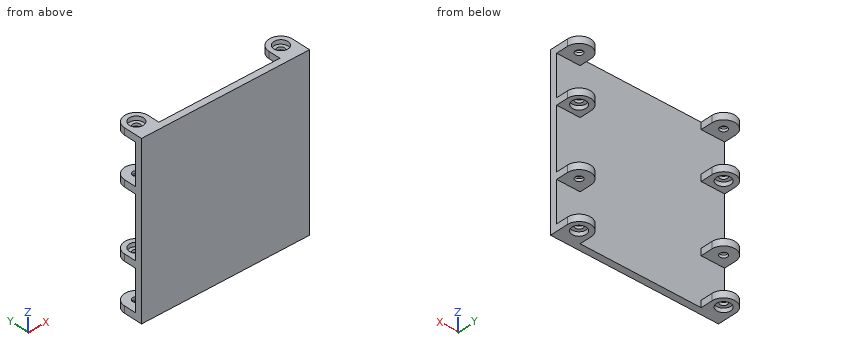
Autodesk Inventor part; units mm, degrees
ref_plane "Work Plane1" through (0, 0, 90) normal (0, 0, 1) x (1, 0, 0)
ref_plane "Work Plane2" through (0, 0, -90) normal (0, 0, 1) x (1, 0, 0)
ref_plane "YZ Plane" through (0, 0, 0) normal (1, 0, 0) x (0, 1, 0)
sketch "Sketch1" plane through (0, 0, 0) normal (0, 0, 1) x (1, 0, 0)
  line L0 (-250, -10) -> (250, -10)
  line L1 (250, -10) -> (250, 10)
  line L2 (250, 10) -> (-250, 10)
  line L3 (-250, 10) -> (-250, -10)
  line L4 (-250, -10) -> (250, 10) construction
  line L5 (250, -10) -> (-250, 10) construction
  point P0 (0, 0)
  dimension "d0" = 500
  dimension "d1" = 20
extrude "Extrusion1" add sketch "Sketch1" along normal mid plane 500
sketch "Sketch2" plane through (0, 0, 250) normal (0, 0, 1) x (1, 0, 0)
  arc A0 (-180, 45) -> (-250, 45) centre (-215, 45) ccw
  line L0 (250, 10) -> (-250, 10) construction
  circle A1 centre (-215, 45) radius 11
  line L1 (-250, 45) -> (-250, 0)
  line L2 (-180, 45) -> (-180, 0)
  line L3 (-180, 0) -> (-250, 0)
  point P0 (0, 0)
  dimension "d4" = 70
  dimension "d5" = 215
  dimension "d6" = 45
  dimension "d7" = 22
  dimension "d9" = 10
extrude "Extrusion2" add sketch "Sketch2" against normal blind 20
ref_plane "Work Plane1" through (0, 0, 90) normal (0, 0, 1) x (1, 0, 0)
sketch "Sketch3" plane through (0, 0, 90) normal (0, 0, 1) x (1, 0, 0)
  arc A0 (-180, 45) -> (-250, 45) centre (-215, 45) ccw construction
  circle A1 centre (-215, 45) radius 11 construction
  line L0 (-180, 45) -> (-180, 10) construction
  line L1 (-250, 45) -> (-250, -10) construction
  circle A2 centre (-215, 45) radius 11
  arc A3 (-180, 45) -> (-250, 45) centre (-215, 45) ccw
  line L2 (-250, 45) -> (-250, 0)
  line L3 (-180, 45) -> (-180, 0)
  line L4 (-180, 0) -> (-250, 0)
  point P0 (0, 0)
extrude "Extrusion3" add sketch "Sketch3" along normal blind 20
sketch "Sketch4" plane through (0, 0, 250) normal (0, 0, 1) x (1, 0, 0)
  circle A0 centre (-215, 45) radius 11 construction
  circle A1 centre (-215, 45) radius 21
  point P0 (0, 0)
  dimension "d15" = 42
extrude "Extrusion4" cut sketch "Sketch4" against normal blind 12
sketch "Sketch5" plane through (0, 0, 90) normal (0, 0, -1) x (-1, 0, 0)
  circle A0 centre (215, 45) radius 11 construction
  circle A1 centre (215, 45) radius 21
  point P0 (0, 0)
  dimension "d18" = 42
extrude "Extrusion5" cut sketch "Sketch5" against normal blind 12
sketch "Sketch6" plane through (0, 0, 250) normal (0, 0, 1) x (1, 0, 0)
  arc A0 (250, 45) -> (180, 45) centre (215, 45) ccw
  circle A1 centre (215, 45) radius 11
  line L0 (180, 45) -> (180, 0)
  line L1 (180, 0) -> (250, 0)
  line L2 (250, 0) -> (250, 45)
  point P0 (0, 0)
  dimension "d21" = 70
  dimension "d22" = 215
  dimension "d23" = 45
  dimension "d24" = 22
  dimension "d25" = 0
extrude "Extrusion6" add sketch "Sketch6" against normal blind 20
sketch "Sketch7" plane through (0, 0, 90) normal (0, 0, 1) x (1, 0, 0)
  arc A0 (250, 45) -> (180, 45) centre (215, 45) ccw construction
  circle A1 centre (215, 45) radius 11 construction
  arc A2 (250, 45) -> (180, 45) centre (215, 45) ccw
  circle A3 centre (215, 45) radius 11
  circle A4 centre (215, 45) radius 11
  line L0 (250, 45) -> (250, 10)
  line L1 (250, 45) -> (250, 0)
  line L2 (250, 0) -> (250, 0)
  arc A5 (250, 45) -> (180, 45) centre (215, 45) ccw
  line L3 (250, 0) -> (250, 45)
  line L4 (180, 45) -> (180, 0)
  line L5 (180, 0) -> (250, 0)
  point P0 (0, 0)
  dimension "d28" = 22
  dimension "d29" = 45
extrude "Extrusion7" add sketch "Sketch7" along normal blind 20
sketch "Sketch8" plane through (0, 0, 250) normal (0, 0, 1) x (1, 0, 0)
  circle A0 centre (215, 45) radius 11 construction
  circle A1 centre (215, 45) radius 21
  point P0 (0, 0)
  dimension "d32" = 42
extrude "Extrusion8" cut sketch "Sketch8" against normal blind 12
sketch "Sketch9" plane through (0, 0, 90) normal (0, 0, -1) x (-1, 0, 0)
  circle A0 centre (-215, 45) radius 11 construction
  circle A1 centre (-215, 45) radius 21
  point P0 (0, 0)
  dimension "d35" = 42
extrude "Extrusion9" cut sketch "Sketch9" against normal blind 12
sketch "Sketch10" plane through (0, 0, -250) normal (0, 0, -1) x (-1, 0, 0)
  arc A0 (-180, 45) -> (-250, 45) centre (-215, 45) ccw construction
  line L0 (-180, 45) -> (-180, 10) construction
  line L1 (-250, 10) -> (-250, 45) construction
  line L2 (250, 10) -> (-250, 10) construction
  circle A1 centre (-215, 45) radius 11 construction
  arc A2 (-180, 45) -> (-250, 45) centre (-215, 45) ccw
  arc A3 (-180, 45) -> (-250, 45) centre (-215, 45) ccw
  circle A4 centre (-215, 45) radius 11
  line L3 (-250, 45) -> (-250, 10)
  line L4 (-250, -10) -> (-250, 45) construction
  line L5 (-180, 10) -> (-180, 45)
  line L6 (-250, 10) -> (-180, 10)
  point P0 (0, 0)
  dimension "d38" = 22
extrude "Extrusion10" add sketch "Sketch10" against normal blind 20
sketch "Sketch11" plane through (0, 0, -250) normal (0, 0, -1) x (-1, 0, 0)
  arc A0 (250, 45) -> (180, 45) centre (215, 45) ccw construction
  circle A1 centre (215, 45) radius 11 construction
  arc A2 (250, 45) -> (180, 45) centre (215, 45) ccw
  arc A3 (250, 45) -> (180, 45) centre (215, 45) ccw
  circle A4 centre (215, 45) radius 11
  line L0 (180, 45) -> (180, 10)
  line L1 (180, 10) -> (250, 10)
  line L2 (180, 45) -> (180, 10)
  line L3 (180, 10) -> (250, 10)
  line L4 (250, 10) -> (250, 45)
  point P0 (0, 0)
  dimension "d41" = 22
extrude "Extrusion11" add sketch "Sketch11" against normal blind 20
ref_plane "Work Plane2" through (0, 0, -90) normal (0, 0, 1) x (1, 0, 0)
sketch "Sketch12" plane through (0, 0, -90) normal (0, 0, 1) x (1, 0, 0)
  arc A0 (250, 45) -> (180, 45) centre (215, 45) ccw construction
  circle A1 centre (215, 45) radius 11 construction
  arc A2 (250, 45) -> (180, 45) centre (215, 45) ccw
  arc A3 (250, 45) -> (180, 45) centre (215, 45) ccw
  circle A4 centre (215, 45) radius 11
  line L0 (250, 10) -> (180, 10)
  line L1 (250, 45) -> (250, 10)
  line L2 (250, 10) -> (180, 10)
  line L3 (180, 10) -> (180, 45)
  point P0 (0, 0)
extrude "Extrusion12" add sketch "Sketch12" against normal blind 20
sketch "Sketch13" plane through (0, 0, -250) normal (0, 0, -1) x (-1, 0, 0)
  circle A0 centre (-215, 45) radius 11 construction
  circle A1 centre (-215, 45) radius 21
  point P0 (0, 0)
  dimension "d47" = 42
extrude "Extrusion13" cut sketch "Sketch13" against normal blind 12
sketch "Sketch14" plane through (0, 0, -90) normal (0, 0, 1) x (1, 0, 0)
  circle A0 centre (215, 45) radius 11 construction
  circle A1 centre (215, 45) radius 21
  point P0 (0, 0)
  dimension "d50" = 42
extrude "Extrusion14" cut sketch "Sketch14" against normal blind 12
sketch "Sketch15" plane through (0, 0, -90) normal (0, 0, 1) x (1, 0, 0)
  arc A0 (-180, 45) -> (-250, 45) centre (-215, 45) ccw
  arc A1 (-180, 45) -> (-250, 45) centre (-215, 45) ccw
  arc A2 (-180, 45) -> (-250, 45) centre (-215, 45) ccw construction
  circle A3 centre (-215, 45) radius 11 construction
  circle A4 centre (-215, 45) radius 11
  line L0 (-180, 45) -> (-180, 10)
  line L1 (-180, 45) -> (-180, 10)
  line L2 (-250, 10) -> (-180, 10)
  line L3 (-180, 10) -> (-250, 10)
  line L4 (-250, 10) -> (-250, 45)
  point P0 (0, 0)
  dimension "d53" = 22
extrude "Extrusion15" add sketch "Sketch15" against normal blind 20
sketch "Sketch16" plane through (0, 0, -250) normal (0, 0, -1) x (-1, 0, 0)
  circle A0 centre (215, 45) radius 11 construction
  circle A1 centre (215, 45) radius 21
  point P0 (0, 0)
  dimension "d56" = 42
extrude "Extrusion16" cut sketch "Sketch16" against normal blind 12
sketch "Sketch17" plane through (0, 0, -90) normal (0, 0, 1) x (1, 0, 0)
  circle A0 centre (-215, 45) radius 11 construction
  circle A1 centre (-215, 45) radius 21
  point P0 (0, 0)
  dimension "d59" = 42
extrude "Extrusion17" cut sketch "Sketch17" against normal blind 12
properties part number "MecanumPlate_FEA" material "Aluminum 6061"
Geometry: final body of the model. Coordinates: model frame, mm. Coordinates: 2 decimals unless noted, no trailing zeros. Order: outer loops, then holes, each group sorted by start corner. A loop starts at its lowest first (then second) coordinate and runs counter-clockwise, first axis right, second up. Notation, with made-up numbers: (15, 35) -> (60, 35) arc R24 cw to (60, 45) -> close; hole circle Ø3 at (-37.75, 40). An arc over 180 degrees is marked (long way). Write each question's results on one line, items separated by ' | '. Start each with the question number.
1) Material intervals for line 1 along Z through (x, y) = (196, 19); line 2 along Y through (x, z) = (-215, -236); line 3 along Y through (x, z) = (-215, 247.25), sorted ascending.
2) Cut plane C-C, the plane x = 123. Output: boundary loops of the cut face in (y, z), and give its area (3 significant figures).
3) First-contact query: pin 1 (8 mm diameter, centred on x = 118, z = -64, fed in from +Y); pin 2 (12.5 mm diameter, centred on x = 207.5, y = 43.5, fed in from -Z); pin 3 (12.5 mm diameter, centred on x = 216.5, y = 47.5, fed in from +Z); pin 4 (21 mm diameter, centred on x = -221, y = 43, fed in from +Z). Flat tips, straight axial feed; report the tip coordinate or a pass-through.
4) Cut plane A-A, the plane x = -215. State how many separate pieces and enclosed holes the cut face has, and give its area (3 significant figures).
5) Cut plane B-B, the plane z = -141. Output: boundary loops of the cut face in (x, y), and give its area (3 significant figures).
Checks:
1) line 1: -250 to -230, -110 to -90, 90 to 110, 230 to 250 | line 2: -10 to 34, 56 to 80 | line 3: -10 to 24, 66 to 80
2) outline: (-10, -250) -> (10, -250) -> (10, 250) -> (-10, 250) -> close | area: 10,000 mm^2
3) pin 1: y = 10 | pin 2: z = -238 | pin 3: through | pin 4: z = 238
4) separate pieces: 5 | enclosed holes: 0 | area: 12,900 mm^2
5) outline: (-250, -10) -> (250, -10) -> (250, 10) -> (-250, 10) -> close | area: 10,000 mm^2
